```python
from build123d import *

# Parameters (mm, degrees)
SKETCH_1_W          = 76
SKETCH_1_H          = 53
SKETCH_1_R          = 1.55
EXTRUDE_1_DEPTH     = 1.5
SKETCH_2_W          = 76
SKETCH_2_H          = 1.5
EXTRUDE_2_DEPTH     = 1.5
SKETCH_3_W          = 76
SKETCH_3_H          = 1.5
EXTRUDE_3_DEPTH     = 35.02
SKETCH_4_R          = 5.36
SKETCH_4_R_2        = 2.600000007
CUT_EXTRUDE_1_DEPTH = 60
SKETCH_5_R          = 2.05
CUT_EXTRUDE_2_DEPTH = 10


with BuildPart() as part:
    # 草图1 → 凸台-拉伸1 (new body)
    with BuildSketch(Plane(origin=(0, 0, 0), x_dir=(1, 0, 0), z_dir=(0, 1, 0))):
        Rectangle(SKETCH_1_W, SKETCH_1_H)
        with Locations((-34.29, 22.86)):
            Circle(SKETCH_1_R, mode=Mode.SUBTRACT)
        with Locations((-34.29, -22.86)):
            Circle(SKETCH_1_R, mode=Mode.SUBTRACT)
        with Locations((34.29, -22.86)):
            Circle(SKETCH_1_R, mode=Mode.SUBTRACT)
        with Locations((34.29, 22.86)):
            Circle(SKETCH_1_R, mode=Mode.SUBTRACT)
    extrude(amount=EXTRUDE_1_DEPTH)

    # 草图2 → 凸台-拉伸2 (add)
    with BuildSketch(Plane.XY.offset(26.5)):
        with Locations((0, 0.75)):
            Rectangle(SKETCH_2_W, SKETCH_2_H)
    extrude(amount=EXTRUDE_2_DEPTH)

    # 草图3 → 凸台-拉伸3 (add)
    with BuildSketch(Plane(origin=(0, 1.5, 0), x_dir=(1, 0, 0), z_dir=(0, 1, 0))):
        with Locations((0, -27.25)):
            Rectangle(SKETCH_3_W, SKETCH_3_H)
    extrude(amount=EXTRUDE_3_DEPTH)

    # 草图4 → 切除-拉伸1 (cut)
    with BuildSketch(Plane(origin=(0, 0, 26.5), x_dir=(-1, 0, 0), z_dir=(0, 0, -1))):
        with Locations((0, 19.02)):
            Circle(SKETCH_4_R)
        with Locations((-12.7, 19.02)):
            Circle(SKETCH_4_R_2)
        with Locations((-25.4, 19.02)):
            Circle(SKETCH_4_R_2)
        with Locations((12.7, 19.02)):
            Circle(SKETCH_4_R_2)
        with Locations((25.4, 19.02)):
            Circle(SKETCH_4_R_2)
    extrude(amount=-CUT_EXTRUDE_1_DEPTH, mode=Mode.SUBTRACT)

    # 草图5 → 切除-拉伸2 (cut)
    with BuildSketch(Plane(origin=(0, 0, 26.5), x_dir=(-1, 0, 0), z_dir=(0, 0, -1))):
        with Locations((-35, 33.52)):
            Circle(SKETCH_5_R)
        with Locations((-35, 5.5)):
            Circle(SKETCH_5_R)
        with Locations((35, 5.5)):
            Circle(SKETCH_5_R)
        with Locations((35, 33.52)):
            Circle(SKETCH_5_R)
    extrude(amount=-CUT_EXTRUDE_2_DEPTH, mode=Mode.SUBTRACT)


solid = part.part
```
Could you check a few things on this model? Use its own coordinates, in mm. A direction names the side the tool comes from. Coordinates: 2 decimals unless noted, no trailing zeros. Write each loop counter-clockwise with the first axis right and the second up, starting at its lowest first coordinate (ties: lowest second). Pieces come first, ordered by that corner, then holes. Notation, with made-up numbers: M 78.25,67.5 L 118.25,67.5 A15 ccw 118.25,86.5 Z; hole C 0,88.5 d5. An arc over 180 degrees is marked long. Answer as CSV lines item,"result". Start each with the question number.
1) For faces 1 (the flat face through (-1, 11, 26.5)), 2 (the cylindrical face through (35.005, 0.74, -21.485)), which set-ups out of +Z, -Z, +X, -X, +Y, -Y let a thin tool reach every point of the face, with its end or its side?
2) Please list where these lines run through material, in increasing order: line 1 (Z direction, x = -34.29, y = 0.85); line 2 (Y direction, x = -35, z = 27.5); line 3 (X direction, y = 5, z = 27). Write a range as from..to.
3) I want a section at D-D, the plane y = 19.02. Please give me the cut outline in (x, z), and give its area (3 significant figures).
4) For P1, Ø4, axis at x = -34.29, z = 22.86, coming from the -Y side; P2, Ø8, axis at x = 8.5, y = 29.5, coming from the -Z side; P3, Ø6, axis at x = -12, z = 0, coming from the +Y side, each with a flat end and sliding along its axis, tell me the tip position at first contact or that it passes through.
5) We'd pull the mould along Y, two halves only. Please class faces 3 (the flat face through (38, 1, 13)), 4 (the cylindrical face through (13.26, 16.48, 27.24)), 5 (the flat face through (-1, 0, 0)), 6 (the cylindrical face through (-23.337, 17.438, 27.24)): +Y half, -Y half, draft (parallel to the pull), parting line (faces both ways), or undercut.
6) I want a section at A-A, the plane z = -22.86. Please give me the cut outline in (x, y).
7) I want a section at B-B, the plane y = 5.5. Please give me the cut outline in (x, z), and give its area (3 significant figures).
8) I want a section at C-C, the plane x = 25.4. Please give me the cut outline in (y, z).
Data:
1,face 1,"-Z, +X, -X, +Y"
1,face 2,"+Y, -Y"
2,line 1,"z = -26.5..-24.41, -21.31..21.31, 24.41..28"
2,line 2,"y = 0..3.45, 7.55..31.47, 35.57..36.52"
2,line 3,"x = -38..-36.99, -33.01..33.01, 36.99..38"
3,outline,"M -38,26.5 L -28,26.5 L -28,28 L -38,28 Z; M -22.8,26.5 L -15.3,26.5 L -15.3,28 L -22.8,28 Z; M -10.1,26.5 L -5.36,26.5 L -5.36,28 L -10.1,28 Z; M 5.36,26.5 L 10.1,26.5 L 10.1,28 L 5.36,28 Z; M 15.3,26.5 L 22.8,26.5 L 22.8,28 L 15.3,28 Z; M 28,26.5 L 38,26.5 L 38,28 L 28,28 Z"
3,area,"66.7 mm^2"
4,P1,"stops at y = 0"
4,P2,"stops at z = 26.5"
4,P3,"stops at y = 1.5"
5,face 3,"draft"
5,face 4,"undercut"
5,face 5,"-Y half"
5,face 6,"undercut"
6,outline,"M -38,0 L -35.84,0 L -35.84,1.5 L -38,1.5 Z; M -32.74,0 L 32.74,0 L 32.74,1.5 L -32.74,1.5 Z; M 35.84,0 L 38,0 L 38,1.5 L 35.84,1.5 Z"
7,outline,"M -38,26.5 L -37.05,26.5 L -37.05,28 L -38,28 Z; M -32.95,26.5 L 32.95,26.5 L 32.95,28 L -32.95,28 Z; M 37.05,26.5 L 38,26.5 L 38,28 L 37.05,28 Z"
7,area,"102 mm^2"
8,outline,"M 0,-26.5 L 1.5,-26.5 L 1.5,26.5 L 16.42,26.5 L 16.42,28 L 0,28 Z; M 21.62,26.5 L 36.52,26.5 L 36.52,28 L 21.62,28 Z"
